from build123d import *

# Parameters (mm, degrees)
F0_W      = 300
F0_H      = 300
F1_DEPTH  = 16
F1_TAPER  = 10
F2_W      = 270
F2_H      = 270
F3_DEPTH  = 16
F3_TAPER  = 10
F4_W      = 240
F4_H      = 240
F5_DEPTH  = 16
F5_TAPER  = 10
F6_W      = 210
F6_H      = 210
F7_DEPTH  = 16
F7_TAPER  = 10
F8_W      = 180
F8_H      = 180
F9_DEPTH  = 16
F9_TAPER  = 10
F10_W     = 150
F10_H     = 150
F11_DEPTH = 16
F11_TAPER = 10
F12_W     = 120
F12_H     = 120
F13_DEPTH = 16
F13_TAPER = 10
F14_W     = 90
F14_H     = 90
F15_DEPTH = 16
F15_TAPER = 10
F16_W     = 60
F16_H     = 60
F17_DEPTH = 16
F17_TAPER = 10
F18_W     = 127.5
F18_H     = 45
F18_W_2   = 45
F18_H_2   = 127.5
F19_DEPTH = 144.001
F24_W     = 215.8472527365
F24_H     = 45
F25_DEPTH = 25
F35_DEPTH = 172.501
F36_W     = 45
F36_H     = 215.8472527365
F37_DEPTH = 25
F39_DEPTH = 172.501
F40_W     = 45
F40_H     = 16.4101098933
F41_DEPTH = 144.001
F42_W     = 45
F42_H     = 215.8472527365
F43_DEPTH = 25
F44_W     = 215.8472527365
F44_H     = 45
F45_DEPTH = 25
F47_DEPTH = 210.501
F49_DEPTH = 210.501
F51_DEPTH = 144.001
F52_W     = 2.6628427036
F52_H     = 45
F53_DEPTH = 144.001
F54_W     = 45
F54_H     = 2.6628427036
F54_H_2   = 45
F54_W_2   = 2.6628427036
F55_DEPTH = 144
F57_W     = 45
F57_H     = 45
F58_DEPTH = 16
F59_W     = 47
F59_H     = 47
F60_DEPTH = 16
F61_W     = 10
F61_H     = 12
F62_DEPTH = 210.501
F61_W_2   = 5
F63_DEPTH = 10
F64_W     = 10
F64_H     = 12
F65_DEPTH = 210.501


with BuildPart() as f1:
    # F0 (on Top) → F1 (new body)
    with BuildSketch(Plane.XY):
        Rectangle(F0_W, F0_H)
    extrude(amount=F1_DEPTH, taper=F1_TAPER)

    # F2 (on face) → F3 (join)
    with BuildSketch(Plane.XY.offset(16)):
        Rectangle(F2_W, F2_H)
    extrude(amount=F3_DEPTH, taper=F3_TAPER)

    # F4 (on face) → F5 (join)
    with BuildSketch(Plane.XY.offset(32)):
        Rectangle(F4_W, F4_H)
    extrude(amount=F5_DEPTH, taper=F5_TAPER)

    # F6 (on face) → F7 (join)
    with BuildSketch(Plane.XY.offset(48)):
        Rectangle(F6_W, F6_H)
    extrude(amount=F7_DEPTH, taper=F7_TAPER)

    # F8 (on face) → F9 (join)
    with BuildSketch(Plane.XY.offset(64)):
        Rectangle(F8_W, F8_H)
    extrude(amount=F9_DEPTH, taper=F9_TAPER)

    # F10 (on face) → F11 (join)
    with BuildSketch(Plane.XY.offset(80)):
        Rectangle(F10_W, F10_H)
    extrude(amount=F11_DEPTH, taper=F11_TAPER)

    # F12 (on face) → F13 (join)
    with BuildSketch(Plane.XY.offset(96)):
        Rectangle(F12_W, F12_H)
    extrude(amount=F13_DEPTH, taper=F13_TAPER)

    # F14 (on face) → F15 (join)
    with BuildSketch(Plane.XY.offset(112)):
        Rectangle(F14_W, F14_H)
    extrude(amount=F15_DEPTH, taper=F15_TAPER)

    # F16 (on face) → F17 (join)
    with BuildSketch(Plane.XY.offset(128)):
        Rectangle(F16_W, F16_H)
    extrude(amount=F17_DEPTH, taper=F17_TAPER)

    # F18 (on face) → F19 (cut, through all)
    with BuildSketch(Plane.XY.offset(144)):
        with Locations((86.25, 0)):
            Rectangle(F18_W, F18_H)
        Rectangle(F18_W_2, F18_H)
        with Locations((0, 86.25)):
            Rectangle(F18_W_2, F18_H_2)
        with Locations((-86.25, 0)):
            Rectangle(F18_W, F18_H)
        with Locations((0, -86.25)):
            Rectangle(F18_W_2, F18_H_2)
    extrude(amount=-F19_DEPTH, mode=Mode.SUBTRACT)


with BuildPart() as f25:
    # F24 (on 3pt) → F25 (new body)
    with BuildSketch(Plane(origin=(81.002945378, 0, 93.0971351393), x_dir=(0.7544092187, 0, -0.6564043957), z_dir=(0.6564043957, 0, 0.7544092187))):
        with Locations((33.9053067481, 0)):
            Rectangle(F24_W, F24_H)
    extrude(amount=-F25_DEPTH)

    # F34 (on face) → F35 (cut, through all)
    with BuildSketch(Plane(origin=(0, 22.5, 0), x_dir=(-1, 0, 0), z_dir=(0, 1, 0))):
        Polygon((-8.7527328104, 122.822855035), (-22.5, 138.6226655897), (-22.5, 110.8614866041), align=None)
        Polygon((-171.5898901067, -18.8602304676), (-149.9137224513, 0), (-188, 0), align=None)
    extrude(amount=-F35_DEPTH, mode=Mode.SUBTRACT)

    # F52 (on face) → F53 (cut, through all)
    with BuildSketch(Plane.XY.offset(144)):
        with Locations((23.8314213518, 0)):
            Rectangle(F52_W, F52_H)
    extrude(amount=-F53_DEPTH, mode=Mode.SUBTRACT)


with BuildPart() as f37:
    # F36 (on 3pt) → F37 (new body)
    with BuildSketch(Plane(origin=(0, 81.002945378, 93.0971351393), x_dir=(1, 0, 0), z_dir=(0, 0.6564043957, 0.7544092187))):
        with Locations((0, 33.9053067481)):
            Rectangle(F36_W, F36_H)
    extrude(amount=-F37_DEPTH)

    # F38 (on face) → F39 (cut, through all)
    with BuildSketch(Plane.YZ.offset(22.5)):
        Polygon((171.5898901067, -18.8602304676), (188, 0), (149.9137224513, 0), align=None)
    extrude(amount=-F39_DEPTH, mode=Mode.SUBTRACT)

    # F40 (on face) → F41 (cut, through all)
    with BuildSketch(Plane.XY.offset(144)):
        with Locations((0, 16.957787757)):
            Rectangle(F40_W, F40_H)
    extrude(amount=-F41_DEPTH, mode=Mode.SUBTRACT)


with BuildPart() as f43:
    # F42 (on 3pt) → F43 (new body)
    with BuildSketch(Plane(origin=(0, -81.002945378, 93.0971351393), x_dir=(1, 0, 0), z_dir=(0, 0.6564043957, -0.7544092187))):
        with Locations((0, 33.9053067481)):
            Rectangle(F42_W, F42_H)
    extrude(amount=F43_DEPTH)

    # F46 (on face) → F47 (cut, through all)
    with BuildSketch(Plane(origin=(-22.5, 0, 0), x_dir=(0, -1, 0), z_dir=(-1, 0, 0))):
        Polygon((171.5898901067, -18.8602304676), (188, 0), (149.9137224513, 0), align=None)
    extrude(amount=-F47_DEPTH, mode=Mode.SUBTRACT)


with BuildPart() as f45:
    # F44 (on 3pt) → F45 (new body)
    with BuildSketch(Plane(origin=(-81.002945378, 0, 93.0971351393), x_dir=(0.7544092187, 0, 0.6564043957), z_dir=(0.6564043957, 0, -0.7544092187))):
        with Locations((-33.9053067481, 0)):
            Rectangle(F44_W, F44_H)
    extrude(amount=F45_DEPTH)

    # F48 (on face) → F49 (cut, through all)
    with BuildSketch(Plane(origin=(0, 22.5, 0), x_dir=(-1, 0, 0), z_dir=(0, 1, 0))):
        Polygon((171.5898901067, -18.8602304676), (188, 0), (149.9137224513, 0), align=None)
    extrude(amount=-F49_DEPTH, mode=Mode.SUBTRACT)


with BuildPart() as f51_tool:
    # F50 (on face) → F51 (new body, through all)
    with BuildSketch(Plane.XY.offset(144)):
        Polygon((-22.5, -25.1628427036), (22.5, -25.1628427036), (22.5, -8.7527328104), (-8.7527328104, -8.7527328104), (-8.7527328104, 22.5), (-25.1628427036, 22.5), (-25.1628427036, -22.5), (-22.5, -22.5), align=None)
    extrude(amount=-F51_DEPTH)


with BuildPart() as f43_1:
    add(f43.part)

    # F51: cut by f51_tool
    add(f51_tool.part, mode=Mode.SUBTRACT)


with BuildPart() as f45_1:
    add(f45.part)

    # F51: cut by f51_tool
    add(f51_tool.part, mode=Mode.SUBTRACT)


with BuildPart() as f55:
    # F54 (on Top) → F55 (new body)
    with BuildSketch(Plane.XY):
        with Locations((0, -23.8314213518)):
            Rectangle(F54_W, F54_H)
        Rectangle(F54_W, F54_H_2)
        with Locations((23.8314213518, 0)):
            Rectangle(F54_W_2, F54_H_2)
        with Locations((-23.8314213518, 0)):
            Rectangle(F54_W_2, F54_H_2)
        with Locations((0, 23.8314213518)):
            Rectangle(F54_W, F54_H)
    extrude(amount=F55_DEPTH)


with BuildPart() as f1_1:
    add(f1.part)

    # F56: union F25, F43, F45, F55, F37
    add(f25.part)
    add(f43_1.part)
    add(f45_1.part)
    add(f55.part)
    add(f37.part)

    # F57 (on face) → F58 (join)
    with BuildSketch(Plane.XY.offset(144)):
        Rectangle(F57_W, F57_H)
    extrude(amount=F58_DEPTH)

    # F59 (on face) → F60 (join)
    with BuildSketch(Plane.XY.offset(160)):
        Rectangle(F59_W, F59_H)
    extrude(amount=F60_DEPTH)

    # F61 (on face) → F62 (cut, through all)
    with BuildSketch(Plane.XZ.offset(22.5)):
        with Locations((0, 150)):
            Rectangle(F61_W, F61_H)
    extrude(amount=-F62_DEPTH, mode=Mode.SUBTRACT)

    # F61 (on face) → F63 (cut)
    with BuildSketch(Plane.XZ.offset(22.5)):
        with Locations((-10.5, 150)):
            Rectangle(F61_W_2, F61_H)
        with Locations((10.5, 150)):
            Rectangle(F61_W_2, F61_H)
    extrude(amount=-F63_DEPTH, mode=Mode.SUBTRACT)

    # F64 (on face) → F65 (cut, through all)
    with BuildSketch(Plane(origin=(-22.5, 0, 0), x_dir=(0, -1, 0), z_dir=(-1, 0, 0))):
        with Locations((0, 150)):
            Rectangle(F64_W, F64_H)
    extrude(amount=-F65_DEPTH, mode=Mode.SUBTRACT)


solid = f1_1.part
Check sheet for the modelled part. Datum: model origin and axes. Units: mm. A direction names the side the tool comes from. Give positions to 0.01 mm unless a question says otherwise; leave off trailing zeros. Write each loop counter-clockwise with the first axis right and the second up, starting at its lowest first coordinate (ties: lowest second). Pieces come first, ordered by that corner, then holes. Notation, with made-up numbers: (69.25, 15.5) -> (77.25, 15.5) arc R16 cw to (77.25, 32.5) -> close; hole circle Ø3 at (38, -4.75). An arc over 180 degrees is marked (long way). Use one line per item in the form item = value. Start each with the question number.
1. Go/stop test with flat-tipped pins: P1, Ø0.7, axis at y = 41.5, z = 127, coming from the -X side; P2, Ø8, axis at y = -113, z = 26, coming from the +X side; P3, Ø5, axis at x = 43.5, y = -13.5, coming from the -Z side; P4, Ø12, axis at x = 89, y = 72.5, coming from the -Z side. Record where each tip stops, or that it passes through.
2. Section check B-B (x = 125). Record the cut outline in (y, z).
3. Access from +Z, -Z, +X, -X, +Y, -Y to the whole of each face (thin tool, end or side, straight path). Record for faces 4 (the flat face through (22.5, 126, 45)), 5 (the flat face through (22.5, -61, 31)), 6 (the flat face through (32, -32, 128)), 7 (the flat face through (-64, -58, 96)).
4. Thickness scan on line 1 along Y through (x, z) = (-21.5, 85); line 2 along Y through (x, z) = (-12.5, 51); line 3 along Z through (x, y) = (-70, 53.5). Record the ranges inside material, lowest first. Write a range as from..to.
5. Section check C-C (z = 53.5). Count the separate pieces of the cut face and the enclosed holes in it, and give its area (3 significant figures).
6. Mould release check, pull along Y, two halves, no side actions. Record for faces 1 (the flat face through (-14, -5, 150)), 2 (the flat face through (-43.61, 33.59, 119.89)), 3 (the flat face through (-71.93, 118.61, 39.89)): pulls with the +Y half, pulls with the -Y half, needs draft (parallel to the pull), parting line crosses it, or undercut.
Conclusion:
q1.P1 = -42.42
q1.P2 = 133.94
q1.P3 = 90.41
q1.P4 = 0
q2.outline = (-150, 0) -> (-22.5, 0) -> (-22.5, 21.68) -> (22.5, 21.68) -> (22.5, 0) -> (150, 0) -> (147.18, 16) -> (135, 16) -> (132.18, 32) -> (22.5, 32) -> (22.5, 54.82) -> (-22.5, 54.82) -> (-22.5, 32) -> (-132.18, 32) -> (-135, 16) -> (-147.18, 16) -> close
q3.face_4 = +Z, +X, +Y
q3.face_5 = -Z
q3.face_6 = +Z, +X, -Y
q3.face_7 = +Z, -X, -Y
q4.line_1 = -90.31..-52.22, -25.16..25.16, 52.22..90.31
q4.line_2 = -129.39..-91.3, -25.16..25.16, 91.3..129.39
q4.line_3 = 0..96
q5.separate_pieces = 1
q5.enclosed_holes = 4
q5.area = 35,900 mm²
q6.face_1 = undercut
q6.face_2 = needs draft
q6.face_3 = pulls with the +Y half
